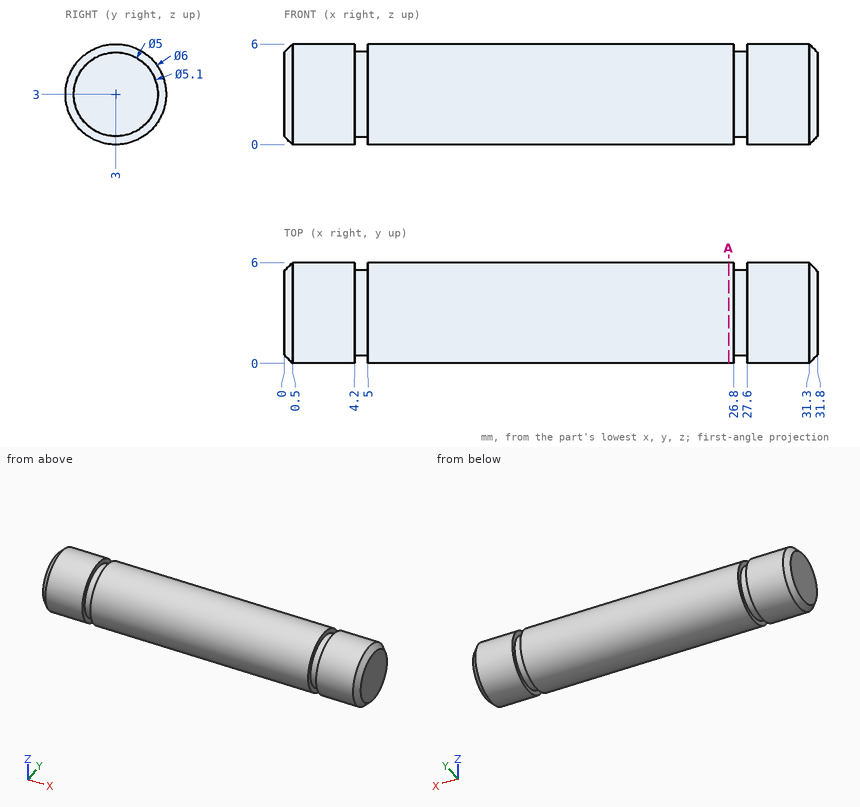
For this review, use the dimensioned drawing (mm, ordinates from the lowest corner) and the shaded views. Coordinates: 2 decimals unless noted, no trailing zeros. Write each loop counter-clockwise with the first axis right and the second up, starting at its lowest first coordinate (ties: lowest second). Pieces come first, ordered by that corner, then holes. Notation, with made-up numbers: (-14.75, -9) - (4.25, -9) arc R11 cw to (4.25, 4) - close; hole circle Ø10 at (-9.75, 0). An arc over 180 degrees is marked (long way). Answer as a JSON object with one key per item and string values. Group by question number.
1. Add section A-A (x = 26.5). Give the boundary of the cut face in (y, z), plus the area to 3 significant figures.
2. To check wall thickness, follow probe 1 along X at (y, z) = (0.8, 1.6); probe 2 along X at (y, z) = (2.5, 5.65); probe 3 along Y at (x, z) = (27, 2.85). State the ranges of each line that lie inside material, in increasing order.
3. Clearance check with a flat-ended pin moving along its axis: pin 1 Ø1.5 at (x, y) = (9, 1) entering from -Z. State where the tip first meets the part, or that it passes through.
Findings:
{
 "1": {"outline": "circle Ø6 at (3, 3)", "area": "28.3 mm²"},
 "2": {"probe 1": "0.11 to 4.2, 5 to 26.8, 27.6 to 31.69", "probe 2": "0.2 to 4.2, 5 to 26.8, 27.6 to 31.6", "probe 3": "0.45 to 5.55"},
 "3": {"pin 1": "z = 0.27"}
}
